Here's how the part is built. I have some questions about the finished solid (model axes, mm). A direction names the side the tool comes from. Round coordinates to 2 decimals unless told otherwise and drop trailing zeros. Write each loop counter-clockwise with the first axis right and the second up, starting at its lowest first coordinate (ties: lowest second). Pieces come first, ordered by that corner, then holes. Notation, with made-up numbers: (40.25, 47) - (51.25, 47) arc R23 cw to (51.25, 62) - close; hole circle Ø2 at (39, 5.5). An arc over 180 degrees is marked (long way). One line per item, written item: value. Start each with the question number.
Item 1: Imagine slicing it at C-C, the plane y = 13.5. Please give me the cut outline in (x, z), then the cut area to 3 significant figures.
Item 2: If I drill on line 1 (X direction, y = 17.3, z = 0); line 2 (X direction, y = 1, z = 0); line 3 (Y direction, x = 11.5, z = 2), over which ranges is the centre line in solid material (lowest first)?
Item 3: Imagine slicing it at A-A, the plane x = 7.5. Please give me the cut outline in (y, z), then the cut area to 3 significant figures.
Item 4: For faces 4 (the face through (6, 16.5, 0)), 5 (the face through (-2, 8, -0.5)), 6 (the face through (-11.09, 8.87, 5.77)), which set-ups out of +Z, -Z, +X, -X, +Y, -Y let a thin tool reach every point of the face, with its end or its side?
Item 5: For P1, Ø5, axis at x = 9.5, z = 2, coming from the -Y side; P2, Ø1.2, axis at x = -2, y = 9.5, coming from the +Z side; P3, Ø1.8, axis at x = 0, z = 0, coming from the +Y side; P4, Ø2.5, axis at x = 6.5, y = 11.5, coming from the +Z side, each with a flat end and sliding along its axis, tell me the tip position at first contact or that it passes through.
Item 6: Imagine slicing it at D-D, the plane x = 0. Please give me the cut outline in (y, z), then the cut area to 3 significant figures.
Item 7: Imagine slicing it at B-B, the plane z = 0. Please give me the cut outline in (x, y).
Item 8: Thinking about a two-plate mould opening in Y: for faces 1 (the face through (-1, 17, 0)), 2 (the face through (-3, 0, 0)), 3 (the face through (6, 1.5, 0)), which applies, released by +Y, released by -Y, zero draft, split by the parting line, or undercut?
```python
from build123d import *

# Parameters (mm, degrees)
SKETCH1_R           = 12.5
BOSS_EXTRUDE1_DEPTH = 18
SKETCH3_R           = 1
CUT_EXTRUDE2_DEPTH  = 26.228951623
SKETCH6_W           = 13
SKETCH6_H           = 15
CUT_EXTRUDE3_DEPTH  = 10
CUT_EXTRUDE4_DEPTH  = 16
SKETCH7_R           = 1
CUT_EXTRUDE5_DEPTH  = 16


with BuildPart() as part:
    # Sketch1 → Boss-Extrude1 (new body)
    with BuildSketch(Plane(origin=(0, 0, 0), x_dir=(1, 0, 0), z_dir=(0, 1, 0))):
        with Locations(Location((0, 0, 0), (0, 0, 270))):
            Circle(SKETCH1_R)
    extrude(amount=BOSS_EXTRUDE1_DEPTH)

    # Sketch3 → Cut-Extrude2 (cut, through all)
    with BuildSketch(Plane.XZ):
        with Locations(Location((7.5, 0, 0), (0, 0, 270))):
            Circle(SKETCH3_R)
    extrude(amount=-CUT_EXTRUDE2_DEPTH, mode=Mode.SUBTRACT)

    # Sketch6 → Cut-Extrude3 (cut)
    with BuildSketch(Plane(origin=(12.5, 0, 0), x_dir=(0, 0, -1), z_dir=(1, 0, 0))):
        with Locations((0, 9)):
            Rectangle(SKETCH6_W, SKETCH6_H)
    extrude(amount=-CUT_EXTRUDE3_DEPTH, mode=Mode.SUBTRACT)

    # Sketch5 → Cut-Extrude4 (cut)
    with BuildSketch(Plane.XZ):
        with BuildLine():
            Line((-1.414213562, 0.5), (-2.514213562, 0.5))
            Line((-2.514213562, 0.5), (-2.514213562, -0.5))
            Line((-2.514213562, -0.5), (-1.414213562, -0.5))
            ThreePointArc((-1.414213562, -0.5), (1.5, 0), (-1.414213562, 0.5))
        make_face()
    extrude(amount=-CUT_EXTRUDE4_DEPTH, mode=Mode.SUBTRACT)

    # Sketch7 → Cut-Extrude5 (cut)
    with BuildSketch(Plane(origin=(0, 18, 0), x_dir=(1, 0, 0), z_dir=(0, 1, 0))):
        with Locations(Location((0, 0, 0), (0, 0, 270))):
            Circle(SKETCH7_R)
    extrude(amount=-CUT_EXTRUDE5_DEPTH, mode=Mode.SUBTRACT)


solid = part.part
```
Values follow:
1. outline: (2.5, -6.5) - (2.5, 6.5) - (10.68, 6.5) arc R12.5 ccw (long way) to (10.68, -6.5) - close; hole (-2.51, -0.5) - (-1.41, -0.5) arc R1.5 ccw (long way) to (-1.41, 0.5) - (-2.51, 0.5) - close
1. area: 360 mm^2
2. line 1: x = -12.5 to -1, 1 to 6.5, 8.5 to 12.5
2. line 2: x = -12.5 to -2.51, 1.5 to 6.5, 8.5 to 12.5
2. line 3: y = 0 to 1.5, 16.5 to 18
3. outline: (0, -10) - (18, -10) - (18, -1) - (16.5, -1) - (16.5, -6.5) - (1.5, -6.5) - (1.5, -1) - (0, -1) - close; (0, 1) - (1.5, 1) - (1.5, 6.5) - (16.5, 6.5) - (16.5, 1) - (18, 1) - (18, 10) - (0, 10) - close
3. area: 159 mm^2
4. face 4: +X
4. face 5: -Y
4. face 6: +Y, -Y
5. P1: stops at y = 0
5. P2: stops at z = 12.42
5. P3: passes through
5. P4: stops at z = 11.34
6. outline: (0, -12.5) - (18, -12.5) - (18, -1) - (16, -1) - (16, -1.5) - (0, -1.5) - close; (0, 1.5) - (16, 1.5) - (16, 1) - (18, 1) - (18, 12.5) - (0, 12.5) - close
6. area: 398 mm^2
7. outline: (-12.5, 0) - (-2.51, 0) - (-2.51, 16) - (-1, 16) - (-1, 18) - (-12.5, 18) - close; (1, 16) - (1.5, 16) - (1.5, 0) - (6.5, 0) - (6.5, 1.5) - (2.5, 1.5) - (2.5, 16.5) - (6.5, 16.5) - (6.5, 18) - (1, 18) - close; (8.5, 0) - (12.5, 0) - (12.5, 1.5) - (8.5, 1.5) - close; (8.5, 16.5) - (12.5, 16.5) - (12.5, 18) - (8.5, 18) - close
8. face 1: zero draft
8. face 2: released by -Y
8. face 3: undercut
